from build123d import *

# Parameters (mm, degrees)
F3_D     = 11.1125
F3_DEPTH = 31.75
F3_TIP   = 3.3385318145
F4_SIZE  = 0.635
F9_D     = 19.9898
F9_DEPTH = 25.4
F9_START = 2.3646856
F9_TIP   = 6.0055418011


with BuildPart() as f1:
    # F0 (on Front) → F1 (revolve)
    with BuildSketch(Plane.XZ):
        Polygon((-15.875, 0), (0, 0), (0, 101.6), (-12.0523, 101.6), (-12.0523, 69.85), (-11.938, 69.85), (-11.938, 26.5810513018), (-11.938, 23.876), (-12.3386533396, 23.876), align=None)
    revolve(axis=Axis((0, 0, 57.15), (0, 0, 1)))

    # F3
    with Locations(Plane.XY.offset(101.6)):
        with Locations((0, 0)):
            Hole(F3_D / 2, depth=F3_DEPTH)
            with Locations((0, 0, -(F3_DEPTH + F3_TIP / 2))):  # 118° drill point
                Cone(0, F3_D / 2, F3_TIP, mode=Mode.SUBTRACT)

    # F4
    f4_edges = [f1.edges().sort_by_distance(p)[0] for p in [
        (12.0523, 0, 101.6),
    ]]
    chamfer(f4_edges, length=F4_SIZE)

    # F5 (on Right) → F6 (revolve)
    with BuildSketch(Plane.YZ):
        with BuildLine():
            Line((0, 0), (0, -1.5446243323))
            ThreePointArc((0, -1.5446243323), (7.9846333239, -1.1575608103), (15.8943893541, 0))
            Line((15.8943893541, 0), (0, 0))
        make_face()
    revolve(axis=Axis((0, 0, -1.5006620425), (0, 0, -1)))

    # F9
    # its depths count from where the whole tool has entered the part; down to there all is cleared
    with Locations(Plane(origin=(0, 0, -3.302), x_dir=(1, 0, 0), z_dir=(0, 0, -1)).offset(-F9_START)):
        with Locations((0, 0)):
            Hole(F9_D / 2, depth=F9_DEPTH)
            with Locations((0, 0, -(F9_DEPTH + F9_TIP / 2))):  # 118° drill point
                Cone(0, F9_D / 2, F9_TIP, mode=Mode.SUBTRACT)


solid = f1.part
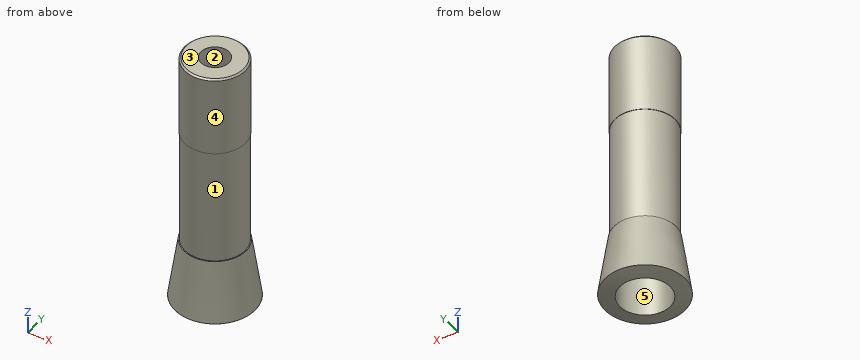
Source: CAD feature listing. Evaluate the final solid. Frame: model axes, mm. Face numbers are marked on the shaded views. A direction names the side the tool comes from. Coordinates: 2 decimals unless noted, no trailing zeros. Loops run counter-clockwise (first coordinate to the right, second up) from the corner with the lowest first, then second, coordinate; pieces in that order, holes last. Notation, with made-up numbers: (29, -11.75) - (79, -11.75) arc R26 cw to (79, 3.25) - close; hole circle Ø6 at (-3.5, -37.5). An arc over 180 degrees is marked (long way). Return JSON: item names as keys, results as strings.
Q1. Section A-A, the plane z = 40. Return loops of the section in (x, y).
Results:
{"outline": "circle Ø23.88 at (0, 0)"}
Q2. Section B-B, the plane z = 29.5. Return loops of the section in (x, y).
Results:
{"outline": "circle Ø23.88 at (0, 0); hole circle Ø3.22 at (0, 0)"}
Q3. Material intervals for line 1 along X through (y, z) = (0, 82); line 2 along Y through (x, z) = (0, 6), sorted ascending.
Results:
{"line 1": "-12.05 to -5.56, 5.56 to 12.05", "line 2": "-14.99 to -9.99, 9.99 to 14.99"}
Q4. Contact query for flat-ended pins moving along their axis: P1, Ø13, axis at x = 0, y = 0, coming from the +Z side; P2, Ø1, axis at x = 9, z = 10, coming from the +Y side; P3, Ø12, axis at y = 9.5, z = 38, coming from the -X side; P4, Ø5, axis at y = -10, z = 21.5, coming from the -X side. Output: stop coordinate, or through.
Results:
{"P1": "z = 101.6", "P2": "y = 11.63", "P3": "x = -11.41", "P4": "x = -10.29"}
Q5. Mould query, pull axis Y, two halves, no side actions, for the marked faces 1, 2 and 3. Classes: released by +Y, released by -Y, zero draft, split by the parting line, or undercut.
Results:
{"face 1": "split by the parting line", "face 2": "undercut", "face 3": "zero draft"}
Q6. Access query for the marked faces 4 and 5. Directions: +Z, -Z, +X, -X, +Y, -Y. A direction counts if a zero-diameter tool reaches every point of the face in a straight line with its end or side. Return the directions, or none.
Results:
{"face 4": "+Z", "face 5": "-Z"}
